Model file for the job. Use its own axes, mm. Face numbers are marked on the shaded views. A direction names the side the tool comes from. Round coordinates to 2 decimals unless told otherwise and drop trailing zeros. Write each loop counter-clockwise with the first axis right and the second up, starting at its lowest first coordinate (ties: lowest second). Pieces come first, ordered by that corner, then holes. Notation, with made-up numbers: (16, -36.75) - (67, -36.75) arc R10 ccw to (67, -23.75) - close; hole circle Ø3 at (52, -11.75). An arc over 180 degrees is marked (long way). One line per item, written item: value.
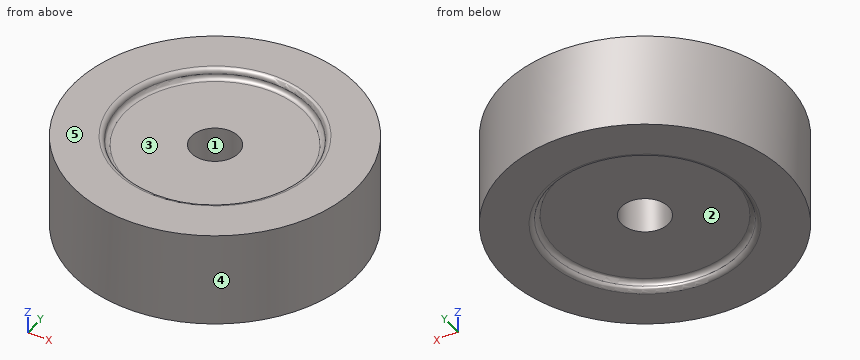
from build123d import *

# Parameters (mm, degrees)
SKETCH1_R           = 30
BOSS_EXTRUDE1_DEPTH = 10
SKETCH2_R           = 20
CUT_EXTRUDE1_DEPTH  = 2
FILLET1_R           = 1
CUT_EXTRUDE2_REACH  = 48.087
SKETCH3_R           = 5


with BuildPart() as part:
    # Sketch1 → Boss-Extrude1 (new, symmetric)
    with BuildSketch(Plane.XY):
        Circle(SKETCH1_R)
    extrude(amount=BOSS_EXTRUDE1_DEPTH, both=True)

    # Sketch2 → Cut-Extrude1 (cut)
    with BuildSketch(Plane.XY.offset(10)):
        Circle(SKETCH2_R)
    cut_extrude1 = extrude(amount=-CUT_EXTRUDE1_DEPTH, mode=Mode.SUBTRACT)

    # Mirror1: Cut-Extrude1 across plane
    add(cut_extrude1.mirror(Plane.XY), mode=Mode.SUBTRACT)

    # Fillet1
    fillet1_edges = [part.edges().sort_by_distance(p)[0] for p in [
        (-20, 0, -10),
        (-20, 0, -8),
        (-20, 0, 8),
        (-20, 0, 10),
    ]]
    fillet(fillet1_edges, radius=FILLET1_R - 0.0001)  # a hair under: the kernel refuses the full size

    # Sketch3 → Cut-Extrude2 (cut, up to next)
    with BuildSketch(Plane.XY.offset(8), mode=Mode.PRIVATE) as cut_extrude2_sk1:
        Circle(SKETCH3_R)
    cut_extrude2_tool1 = extrude(cut_extrude2_sk1.sketch, amount=-CUT_EXTRUDE2_REACH, mode=Mode.PRIVATE) & part.part
    add(cut_extrude2_tool1.solids().sort_by_distance((0, 0, 8))[0], mode=Mode.SUBTRACT)


solid = part.part
1. Tool access for the marked faces 1 and 2: list every direction of +Z, -Z, +X, -X, +Y, -Y with a clear straight run to the whole face (end or side of a thin tool).
Report:
face 1: +Z, -Z
face 2: -Z
2. Mould opens along X. For the marked faces 3, 4 and 5 say: released by +X, released by -X, zero draft, split by the parting line, or undercut.
Report:
face 3: undercut
face 4: split by the parting line
face 5: zero draft
3. Band-saw the part on D-D on y = 26. Write the cut outline in (x, z).
Report:
outline: (-14.97, -10) - (14.97, -10) - (14.97, 10) - (-14.97, 10) - close
4. Drop flat-ended pins along their axis: pin 1 (2 mm diameter, centred on x = -23.5, z = -8, fed in from -Y); pin 2 (4 mm diameter, centred on x = -9, z = 5, fed in from +Y); pin 3 (13 mm diameter, centred on x = 0, y = 0, fed in from +Z). Give the stop position or say it passes through.
Report:
pin 1: y = -19.84
pin 2: y = 29.17
pin 3: z = 8
5. Wall check: probe 1 along Y at (x, z) = (0, 9); probe 2 along Z at (x, y) = (18.5, -2); probe 3 along Y at (x, z) = (0, -3.75). Give the ranges that are in metal, low to high. Write a range as [from, to].
Report:
probe 1: [-30, -20], [20, 30]
probe 2: [-8, 8]
probe 3: [-30, -5], [5, 30]
6. Band-saw the part on C-C on z = 1. Write the cut outline in (x, y).
Report:
outline: circle Ø60 at (0, 0); hole circle Ø10 at (0, 0)
